Check sheet for the drawn part. Datum: minimum x, y, z corner. Units: mm. A direction names the side the tool comes from. Round coordinates to 2 decimals unless told otherwise and drop trailing zeros. Write each loop counter-clockwise with the first axis right and the second up, starting at its lowest first coordinate (ties: lowest second). Pieces come first, ordered by that corner, then holes.
Item 1: Release check for a two-part mould opening along Z. For the marked faces 1, 2, 3 and 4 record: +Z half, -Z half, draft (parallel to the pull), parting line (faces both ways), or undercut.
Item 2: Tool access check on the marked faces 5, 6, 7 and 8. Record the directions out of +Z, -Z, +X, -X, +Y, -Y that give a thin tool (end or side, any length) a straight path to the whole face; none if there is none.
Item 3: Cross-section at B-B on x = 13.75. Enter the section's corners in (y, z).
Item 4: Cross-section at D-D on y = 2.25. Enter the section's corners in (x, z), plus the area to 3 significant figures.
Item 5: Material ranges on line 1 (X direction, y = 5.65, z = 6.5) (3 decimals); line 2 (Z direction, x = 14, y = 2); line 3 (X direction, y = 5.75, z = 7.5), recorded low to high.
Item 6: Cross-section at C-C on z = 3.25. Enter the section's corners in (x, y), plus the area to 3 significant figures.
Item 7: Cross-section at A-A on z = 6.5. Enter the section's corners in (x, y) (3 decimals).
Item 8: Go/stop test with flat-tipped pins: pin 1 Ø1 at (x, y) = (10.5, 1) entering from -Z; pin 2 Ø2 at (x, y) = (24, 5.5) entering from -Z; pin 3 Ø2 at (x, y) = (4, 6.5) entering from +Z. Record where each tip stops, or that it passes through.
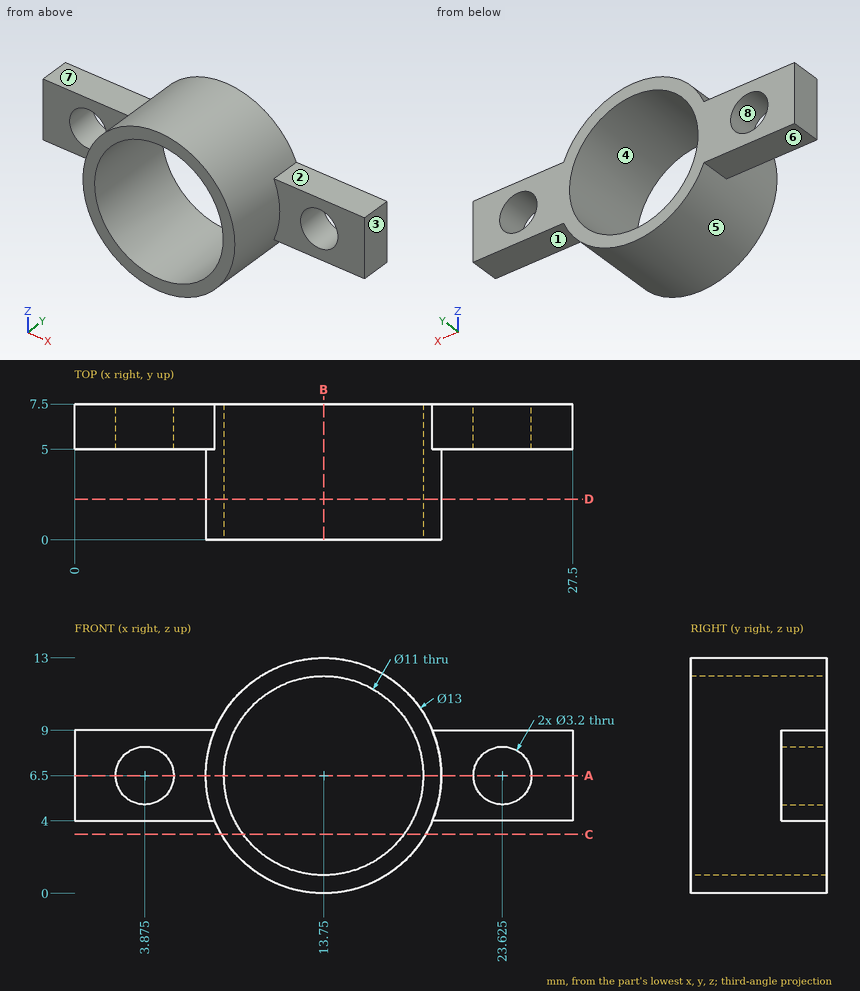
Response values:
1. face 1: -Z half
1. face 2: +Z half
1. face 3: draft
1. face 4: undercut
2. face 5: -Y
2. face 6: -Z, -X, +Y, -Y
2. face 7: +Z, -X, +Y, -Y
2. face 8: +Y, -Y
3. outline: (0, 0) - (7.5, 0) - (7.5, 1) - (0, 1) - close; (0, 12) - (7.5, 12) - (7.5, 13) - (0, 13) - close
4. outline: circle Ø13 at (13.75, 6.5); hole circle Ø11 at (13.75, 6.5)
4. area: 37.7 mm2
5. line 1: x = 0 to 2.275, 5.475 to 8.25, 19.25 to 22.025, 25.225 to 27.5
5. line 2: z = 0 to 1.01, 11.99 to 13
5. line 3: x = 0 to 2.63, 5.12 to 8.34, 19.16 to 22.38, 24.87 to 27.5
6. outline: (8.12, 0) - (9.31, 0) - (9.31, 7.5) - (8.12, 7.5) - close; (18.19, 0) - (19.38, 0) - (19.38, 7.5) - (18.19, 7.5) - close
6. area: 17.9 mm2
7. outline: (0, 5) - (2.275, 5) - (2.275, 7.5) - (0, 7.5) - close; (5.475, 5) - (7.25, 5) - (7.25, 0) - (8.25, 0) - (8.25, 7.5) - (5.475, 7.5) - close; (19.25, 0) - (20.25, 0) - (20.25, 5) - (22.025, 5) - (22.025, 7.5) - (19.25, 7.5) - close; (25.225, 5) - (27.5, 5) - (27.5, 7.5) - (25.225, 7.5) - close
8. pin 1: stops at z = 0.61
8. pin 2: stops at z = 4
8. pin 3: stops at z = 9
